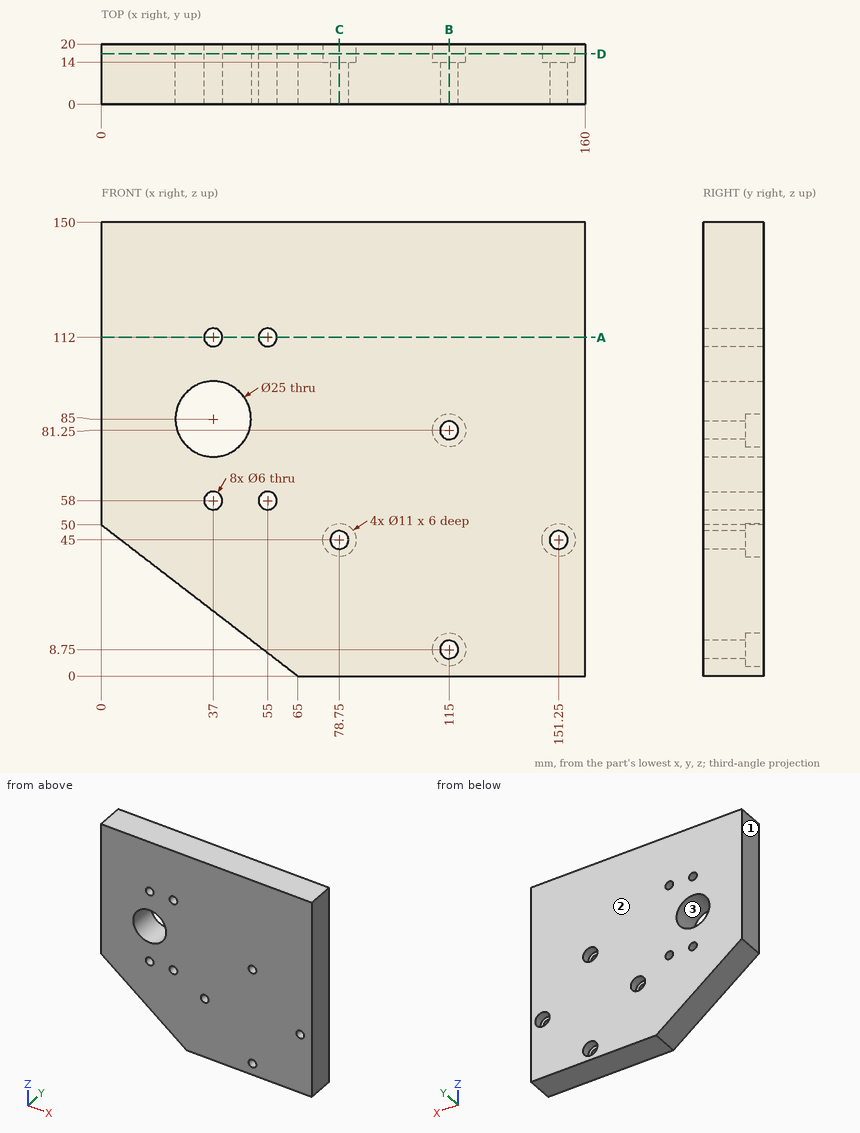
Source: three-view drawing plus pictorial views. Frame: mm from the lowest corner of the part. Coordinates: 2 decimals unless noted, no trailing zeros. Order: outer loops, then holes, each group sorted by start corner. A loop starts at its lowest first (then second) coordinate and runs counter-clockwise, first axis right, second up. Notation, with made-up numbers: M 72,-1 L 98,-1 A20 ccw 98,25 Z; hole C -34.5,77.25 d11. An arc over 180 degrees is marked long. Answer in a Markdown table with one row per item.
(1) Section query A-A, the plane z = 112. Output: boundary loops of the cut face in (x, y), plus the area to 3 significant figures.
Numbers:
| item | result |
|---|---|
| outline | M 0,0 L 34,0 L 34,20 L 0,20 Z; M 40,0 L 52,0 L 52,20 L 40,20 Z; M 58,0 L 160,0 L 160,20 L 58,20 Z |
| area | 2,960 mm^2 |
(2) Contact query for flat-ended pins moving along their axis: pin 1 Ø3.5 at (x, z) = (55, 58) entering from -Y; pin 2 Ø3.5 at (x, z) = (151.5, 43.5) entering from +Y; pin 3 Ø6 at (x, y) = (26, 9.5) entering from -Z. Output: stop coordinate, or through.
Numbers:
| item | result |
|---|---|
| pin 1 | passes through |
| pin 2 | stops at y = 14 |
| pin 3 | stops at z = 27.69 |
(3) Material intervals for line 1 (Z direction, x = 151.25, y = 16.9); line 2 (Z direction, x = 115, y = 8); line 3 (Z direction, x = 78.75, y = 6), sorted ascending. Write a range as [from, to].
Numbers:
| item | result |
|---|---|
| line 1 | z = [0, 39.5], [50.5, 150] |
| line 2 | z = [0, 5.75], [11.75, 78.25], [84.25, 150] |
| line 3 | z = [0, 42], [48, 150] |
(4) Section query D-D, the plane y = 16.75. Give the number of separate pieces and of enclosed holes in the cut face, plus the area to 3 significant figures.
Numbers:
| item | result |
|---|---|
| separate pieces | 1 |
| enclosed holes | 9 |
| area | 21,400 mm^2 |
(5) Draft query along X for the marked faces 1, 2 and 3. Return one class per face: pulls with the +X half, pulls with the -X half, needs draft (parallel to the pull), parting line crosses it, or undercut.
Numbers:
| item | result |
|---|---|
| face 1 | pulls with the -X half |
| face 2 | needs draft |
| face 3 | undercut |
(6) Section query C-C, the plane x = 78.75. Output: boundary loops of the cut face in (y, z).
Numbers:
| item | result |
|---|---|
| outline | M 0,0 L 20,0 L 20,39.5 L 14,39.5 L 14,42 L 0,42 Z; M 0,48 L 14,48 L 14,50.5 L 20,50.5 L 20,150 L 0,150 Z |
(7) Section query B-B, the plane x = 115. Output: boundary loops of the cut face in (y, z), plus the area to 3 significant figures.
Numbers:
| item | result |
|---|---|
| outline | M 0,0 L 20,0 L 20,3.25 L 14,3.25 L 14,5.75 L 0,5.75 Z; M 0,11.75 L 14,11.75 L 14,14.25 L 20,14.25 L 20,75.75 L 14,75.75 L 14,78.25 L 0,78.25 Z; M 0,84.25 L 14,84.25 L 14,86.75 L 20,86.75 L 20,150 L 0,150 Z |
| area | 2,700 mm^2 |
